Check sheet for the drawn part. Datum: minimum x, y, z corner. Units: mm. Give positions to 0.01 mm unless a question says otherwise; leave off trailing zeros. Order: outer loops, then holes, each group sorted by start corner. A loop starts at its lowest first (then second) coordinate and runs counter-clockwise, first axis right, second up. Notation, with made-up numbers: M 33.5,73 L 59.5,73 A10 ccw 59.5,87 Z; hole C 12,-29.5 d11. An arc over 180 degrees is marked long. One line per question, with ' | ' between items. Start each with the question number.
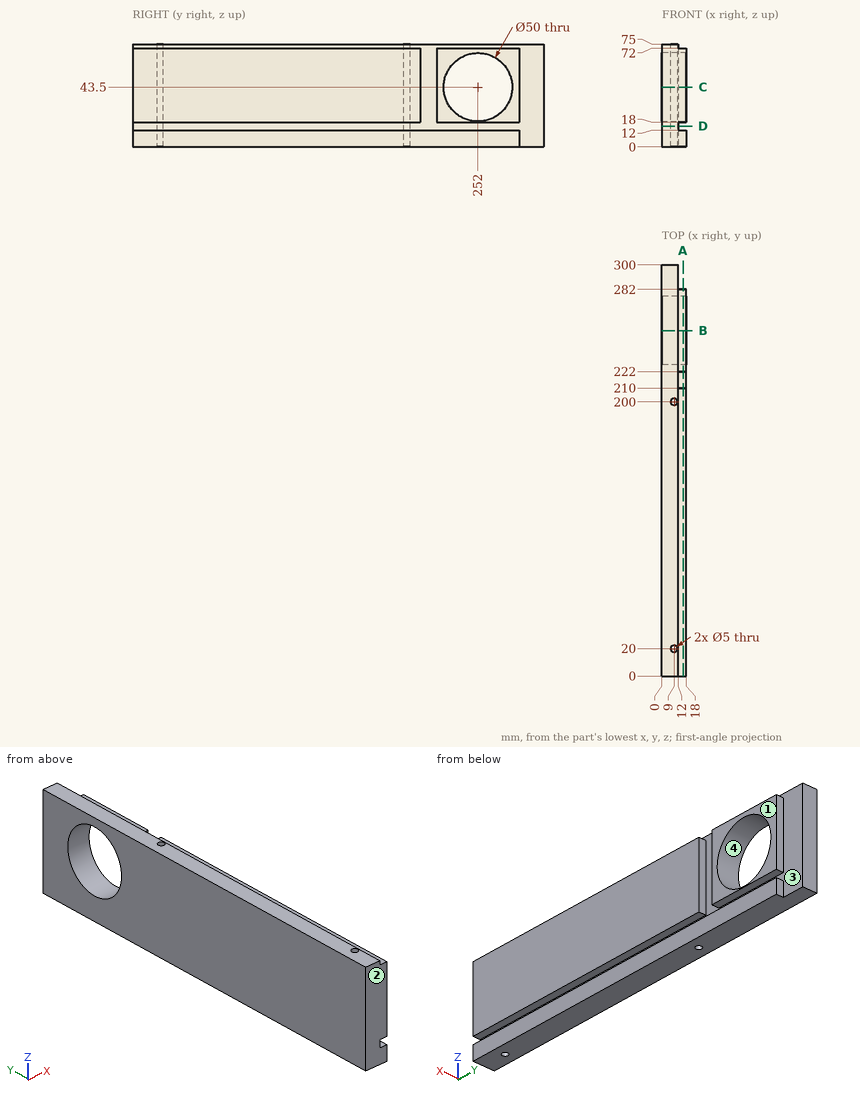
Item 1: Go/stop test with flat-tipped pins: P1, Ø1.8, axis at x = 16, z = 3.5, coming from the +Y side; P2, Ø1.8, axis at x = 15, y = 241, coming from the +Z side. Record where each tip stops, or that it passes through.
Item 2: Section check C-C, the plane z = 43.5. Record the cut outline in (x, y).
Item 3: Scan lines: probe 1 along Y at (x, z) = (9, 42); probe 2 along Y at (x, z) = (9, 13); probe 3 along Y at (x, z) = (7.75, 43.5). Record each from-to range of solid material in increasing order. Write a range as [from, to].
Item 4: Draft check along Y on the marked faces 1, 2, 3 and 4. Enter one of: released by +Y, released by -Y, zero draft, split by the parting line, or undercut.
Item 5: Section check B-B, the plane y = 252. Record the cut outline in (x, z).
Item 6: Section check A-A, the plane x = 15.5. Record the cut outline in (y, z).
Item 7: Section check D-D, the plane z = 15. Record the cut outline in (x, y).
Reported:
1) P1: stops at y = 282 | P2: stops at z = 72
2) outline: M 0,0 L 18,0 L 18,210 L 12,210 L 12,222 L 18,222 L 18,227 L 0,227 Z; M 0,277 L 18,277 L 18,282 L 12,282 L 12,300 L 0,300 Z; hole C 9,20 d5; hole C 9,200 d5
3) probe 1: y = [0, 17.5], [22.5, 197.5], [202.5, 227.05], [276.95, 300] | probe 2: y = [0, 17.5], [22.5, 197.5], [202.5, 300] | probe 3: y = [0, 17.83], [22.17, 197.83], [202.17, 227], [277, 300]
4) face 1: zero draft | face 2: released by -Y | face 3: undercut | face 4: undercut
5) outline: M 0,0 L 18,0 L 18,12 L 12,12 L 12,18 L 18,18 L 18,18.5 L 0,18.5 Z; M 0,68.5 L 18,68.5 L 18,72 L 12,72 L 12,75 L 0,75 Z
6) outline: M 0,0 L 282,0 L 282,12 L 0,12 Z; M 0,18 L 210,18 L 210,72 L 0,72 Z; M 222,18 L 282,18 L 282,72 L 222,72 Z; hole C 252,43.5 d50
7) outline: M 0,0 L 12,0 L 12,300 L 0,300 Z; hole C 9,20 d5; hole C 9,200 d5
